Build history of the part. All positions in model axes, mm. Face numbers are marked on the shaded views. A direction names the side the tool comes from. Give positions to 0.01 mm unless a question says otherwise; leave off trailing zeros. Loops run counter-clockwise (first coordinate to the right, second up) from the corner with the lowest first, then second, coordinate; pieces in that order, holes last. Notation, with made-up numbers: (62.5, 68.25) -> (86.5, 68.25) arc R22 cw to (86.5, 102.25) -> close; hole circle Ø9 at (55, 1). An arc over 180 degrees is marked (long way). One line per question, with ' | ' between items. Start each with the question number.
(1) Slice it at D-D, the plane y = 0. Write the cut outline in (x, z).
(2) Drill centre lines: L1, parallel to Y at x = 0, z = 6.05; L2, parallel to X at y = 0, z = 7; L3, parallel to X at y = -5, z = 7.55. Where is each one in solid material? Low to high. Write a range as from..to.
(3) 3-axis set-ups, long thin cutter, end or side, ignore diameter. For the marked faces 1 and 2: which of +Z, -Z, +X, -X, +Y, -Y reach the whole face in a straight line?
(4) Slice it at B-B, the plane x = -9. Write the cut outline in (y, z), then the cut area to 3 significant figures.
(5) Slice it at C-C, the plane z = 5. Write the cut outline in (x, y), then the cut area to 3 significant figures.
(6) Mould opens along Y. For the marked faces 3, 4 and 5 say: pulls with the +Y half, pulls with the -Y half, needs draft (parallel to the pull), parting line crosses it, or undercut.
(7) Slice it at A-A, the plane y = -5. Write the cut outline in (x, z).
(8) Flat gauge pin, fed straight in: pin 1 Ø2 at (y, z) = (0, 5) entering from -X. Where does the tip first touch, or does it go through?
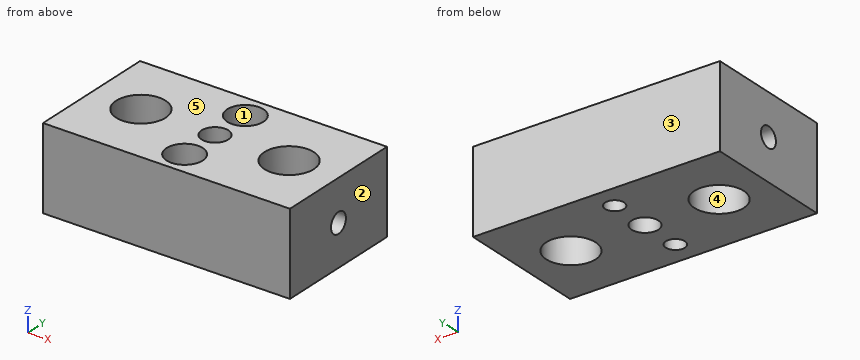
Autodesk Inventor part; units mm, degrees
ref_plane "YZ Plane" through (0, 0, 0) normal (1, 0, 0) x (0, 1, 0)
ref_plane "XZ Plane" through (0, 0, 0) normal (0, 1, 0) x (-1, 0, 0)
ref_plane "XY Plane" through (0, 0, 0) normal (0, 0, 1) x (1, 0, 0)
sketch "Skizze1" plane through (0, 0, 0) normal (0, 0, 1) x (1, 0, 0)
  line L0 (-15, 8) -> (15, 8)
  line L1 (15, 8) -> (15, -8)
  line L2 (15, -8) -> (-15, -8)
  line L3 (-15, -8) -> (-15, 8)
  line L4 (-21, 0) -> (21, 0)
  line L5 (0, -11.2) -> (0, 11.2)
  point P0 (0, 0)
  dimension "d0" = 16
  dimension "d1" = 30
extrude "Extrusion1" add sketch "Skizze1" along normal blind 10
sketch "Skizze2" plane through (0, 0, 10) normal (0, 0, 1) x (1, 0, 0)
  line L0 (-21, 0) -> (21, 0)
  line L1 (0, -11.2) -> (0, 11.2)
  point P0 (0, 0)
  point P1 (-9, 0)
  point P2 (9, 0)
  dimension "d4" = 18
hole "Bohrung1" at (-9, 0, 10) at (9, 0, 10) direction (0, 0, -1) diameter 6 end through all
sketch "Skizze3" plane through (0, 0, 10) normal (0, 0, 1) x (1, 0, 0)
  line L0 (0, -11.2) -> (0, 11.2)
  line L1 (-21, 0) -> (21, 0)
  point P0 (0, 0)
  point P1 (0, 5)
  point P2 (0, -5)
  dimension "d12" = 10
hole "Bohrung2" at (0, 5, 10) at (0, -5, 10) direction (0, 0, -1) diameter 2.3 end through all counterbore diameter 4.4 counterbore depth 6
sketch "Skizze4" plane through (0, 0, 10) normal (0, 0, 1) x (1, 0, 0)
  point P0 (0, 0)
  point P1 (0, 0)
hole "Bohrung3" at (0, 0, 10) direction (0, 0, -1) diameter 3.242 end through all
sketch "Skizze5" plane through (-15, -8, 0) normal (-1, 0, 0) x (0, 0, 1)
  line L0 (10, 0) -> (10, 16)
  line L1 (0, 16) -> (10, 16)
  line L2 (0, 0) -> (10, 0)
  line L3 (0, 8) -> (10, 8)
  line L4 (5, 16) -> (5, 0)
  point P0 (5, 8)
hole "Bohrung4" at (-15, 0, 5) direction (1, 0, 0) diameter 2.459 end up to surface
mirror "Spiegeln1" about plane through (0, 0, 0) normal (1, 0, 0) of "Bohrung4"
properties part number "13_0204_020"
Final values:
1) outline: (-15, 0) -> (-12, 0) -> (-12, 3.77) -> (-15, 3.77) -> close; (-15, 6.23) -> (-12, 6.23) -> (-12, 10) -> (-15, 10) -> close; (-6, 0) -> (-1.62, 0) -> (-1.62, 10) -> (-6, 10) -> close; (1.62, 0) -> (6, 0) -> (6, 10) -> (1.62, 10) -> close; (12, 0) -> (15, 0) -> (15, 3.77) -> (12, 3.77) -> close; (12, 6.23) -> (15, 6.23) -> (15, 10) -> (12, 10) -> close
2) L1: -8..-7.2, -2.8..-1.62, 1.62..2.8, 7.2..8 | L2: -15..-12, -6..-1.62, 1.62..6, 12..15 | L3: -15..-2.2, 2.2..15
3) face 1: +Z | face 2: +Z, -Z, +X, +Y, -Y
4) outline: (-8, 0) -> (-3, 0) -> (-3, 10) -> (-8, 10) -> close; (3, 0) -> (8, 0) -> (8, 10) -> (3, 10) -> close | area: 100 mm2
5) outline: (-15, -8) -> (15, -8) -> (15, -1.23) -> (11.74, -1.23) arc R3 cw (long way) to (11.74, 1.23) -> (15, 1.23) -> (15, 8) -> (-15, 8) -> (-15, 1.23) -> (-11.74, 1.23) arc R3 cw (long way) to (-11.74, -1.23) -> (-15, -1.23) -> close; hole circle Ø4.4 at (0, -5); hole circle Ø4.4 at (0, 5); hole circle Ø3.24 at (0, 0) | area: 370 mm2
6) face 3: pulls with the +Y half | face 4: undercut | face 5: needs draft
7) outline: (-15, 0) -> (-1.15, 0) -> (-1.15, 4) -> (-2.2, 4) -> (-2.2, 10) -> (-15, 10) -> close; (1.15, 0) -> (15, 0) -> (15, 10) -> (2.2, 10) -> (2.2, 4) -> (1.15, 4) -> close
8) pin 1: x = -6.17
